CAD build for the part. Positions are in the model's coordinates, mm. Give positions to 0.01 mm unless a question says otherwise; leave off trailing zeros. Loops run counter-clockwise (first coordinate to the right, second up) from the corner with the lowest first, then second, coordinate; pieces in that order, holes last. Notation, with made-up numbers: (58, -9.5) - (64, -9.5) arc R22 ccw to (64, 12.5) - close; hole circle Ø8 at (40.25, 35.25). An arc over 180 degrees is marked (long way). Return JSON: item names as keys, results as strings.
from build123d import *

# Parameters (mm, degrees)
BOSS_EXTRUDE1_DEPTH = 266.7
CUT_EXTRUDE1_DEPTH  = 304.8
SKETCH3_W           = 204.7875
SKETCH3_H           = 6.35
SKETCH3_H_2         = 133.35
CUT_EXTRUDE2_DEPTH  = 60.706


with BuildPart() as part:
    # Sketch1 → Boss-Extrude1 (new body)
    with BuildSketch(Plane.XY):
        with BuildLine():
            Line((204.7875, -2.511386267), (204.7875, -7.591386267))
            ThreePointArc((204.7875, -7.591386267), (102.270785822, -16.362635969), (0, -5.08))
            Line((0, -5.08), (0, 0))
            ThreePointArc((0, 0), (102.270785822, -11.282635969), (204.7875, -2.511386267))
        make_face()
    extrude(amount=BOSS_EXTRUDE1_DEPTH)

    # Sketch2 → Cut-Extrude1 (cut)
    with BuildSketch(Plane(origin=(0, 0, 0), x_dir=(-1, 0, 0), z_dir=(0, 0, -1))):
        with BuildLine():
            ThreePointArc((0, 0), (-102.270785822, -11.282635969), (-204.7875, -2.511386267))
            Line((-204.7875, -2.511386267), (-204.7875, -3.781386267))
            ThreePointArc((-204.7875, -3.781386267), (-102.270785822, -12.552635969), (0, -1.27))
            Line((0, -1.27), (0, 0))
        make_face()
    extrude(amount=-CUT_EXTRUDE1_DEPTH, mode=Mode.SUBTRACT)

    # Sketch3 → Cut-Extrude2 (cut)
    with BuildSketch(Plane(origin=(0, 0, 0), x_dir=(1, 0, 0), z_dir=(0, 1, 0))):
        with Locations((102.39375, -136.525)):
            Rectangle(SKETCH3_W, SKETCH3_H)
        with Locations((102.39375, -66.675)):
            Rectangle(SKETCH3_W, SKETCH3_H_2)
    extrude(amount=-CUT_EXTRUDE2_DEPTH, mode=Mode.SUBTRACT)


solid = part.part
1. Drill centre lines: probe 1 along Y at (x, z) = (169, 201.5); probe 2 along Y at (x, z) = (60, 184.5). Where is each one in solid material? Low to high.
Values follow:
{"probe 1": "y = -12.95 to -9.14", "probe 2": "y = -14.15 to -10.34"}
2. Cut at C-C, the plane x = 186. Write the cut outline in (y, z).
Values follow:
{"outline": "(-10.72, 139.7) - (-6.91, 139.7) - (-6.91, 266.7) - (-10.72, 266.7) - close"}
3. Cut at B-B, the plane z = 243. Write the cut outline in (x, y).
Values follow:
{"outline": "(0, -5.08) arc R527.87 ccw to (204.79, -7.59) - (204.79, -3.78) arc R527.87 cw to (0, -1.27) - close"}
4. Drop a flat-ended pin along its axis: P1, Ø5, axis at x = 180, z = 218.5, coming from the -Y side. Give the stop position or say it passes through.
Values follow:
{"P1": "stops at y = -11.91"}
